Geometry check sheet. Reference: the model listing, model coordinates, mm. A direction names the side the tool comes from. Round coordinates to 2 decimals unless told otherwise and drop trailing zeros. Loops run counter-clockwise (first coordinate to the right, second up) from the corner with the lowest first, then second, coordinate; pieces in that order, holes last. Notation, with made-up numbers: M 89,-15 L 115,-15 A25 cw 115,-2 Z; hole C 77.5,24 d3. An arc over 180 degrees is marked long. Use one line per item in the form item = value. Start each with the question number.
1. Cross-section at C-C (z = -3.5). Record the boundary of the cut face in (x, y), then the cut area to 3 significant figures.
2. Go/stop test with flat-tipped pins: pin 1 (4 mm diameter, centred on x = 11.5, z = -8, fed in from +Y); pin 2 (6.5 mm diameter, centred on x = 12, y = -10, fed in from +Z); pin 3 (5 mm diameter, centred on y = -11, z = -3.5, fed in from +X). Record where each tip stops, or that it passes through.
3. Cross-section at B-B (y = -15.5). Record the boundary of the cut face in (x, z), then the cut area to 4 significant figures.
4. Set-up check for faces 1 (the flat face through (10, -13, -7.5)), 2 (the flat face through (18, -16, -5)), 3 (the flat face through (10, -13, -2.5)): record each of +Z, -Z, +X, -X, +Y, -Y from which the full face is reachable in a straight line by a thin tool's end or side.
5. Cross-section at A-A (x = 13). Record the boundary of the cut face in (y, z), then the cut area to 3 significant figures.
6. Material ranges on line 1 (Y direction, x = 19.25, z = -8); line 2 (X direction, y = -7.5, z = -3.5); line 3 (Z direction, x = 9, y = -11.5), recorded low to high.
7. Cross-section at D-D (y = -7.5). Record the boundary of the cut face in (x, z), then the cut area to 3 significant figures.
```python
from build123d import *

# Parameters (mm, degrees)
EXTRUDE_1_DEPTH  = 10
RIB_29_REACH     = 33.639
SKETCH_20_WALL_W = 76.590876578
SKETCH_20_WALL_H = 5


with BuildPart() as part:
    # 草图4 → 凸台-拉伸1 (new body)
    with BuildSketch(Plane.XY):
        Polygon((0, 0), (0, -20), (24, -20), (24, -16), (8, -16), (8, 0), align=None)
    extrude(amount=-EXTRUDE_1_DEPTH)

    # 草图20 wall → 筋29 (add, up to next)
    with BuildSketch(Plane(origin=(12, -12, -5), x_dir=(0.707106781187, -0.707106781187, 0), z_dir=(0.707106781187, 0.707106781187, 0)), mode=Mode.PRIVATE) as rib_29_sk1:
        Rectangle(SKETCH_20_WALL_W, SKETCH_20_WALL_H)
    rib_29_tool1 = extrude(rib_29_sk1.sketch, amount=-RIB_29_REACH, mode=Mode.PRIVATE) - part.part
    add(rib_29_tool1.solids().sort_by_distance((12, -12, -5))[0])


solid = part.part
```
Reported:
q1.outline = M 0,-20 L 24,-20 L 24,-16 L 16,-16 L 8,-8 L 8,0 L 0,0 Z
q1.area = 256 mm²
q2.pin_1 = -9.56
q2.pin_2 = -2.5
q2.pin_3 = 13.5
q3.outline = M 0,-10 L 8,-10 L 8,-7.5 L 15.5,-7.5 L 15.5,-2.5 L 8,-2.5 L 8,0 L 0,0 Z
q3.area = 117.5 mm²
q4.face_1 = -Z, +X, +Y
q4.face_2 = +X, +Y
q4.face_3 = +Z, +X, +Y
q5.outline = M -20,-10 L -16,-10 L -16,-7.5 L -13,-7.5 L -13,-2.5 L -16,-2.5 L -16,0 L -20,0 Z
q5.area = 55.0 mm²
q6.line_1 = -20 to -16
q6.line_2 = 0 to 8
q6.line_3 = -7.5 to -2.5
q7.outline = M 0,-10 L 8,-10 L 8,0 L 0,0 Z
q7.area = 80.0 mm²
